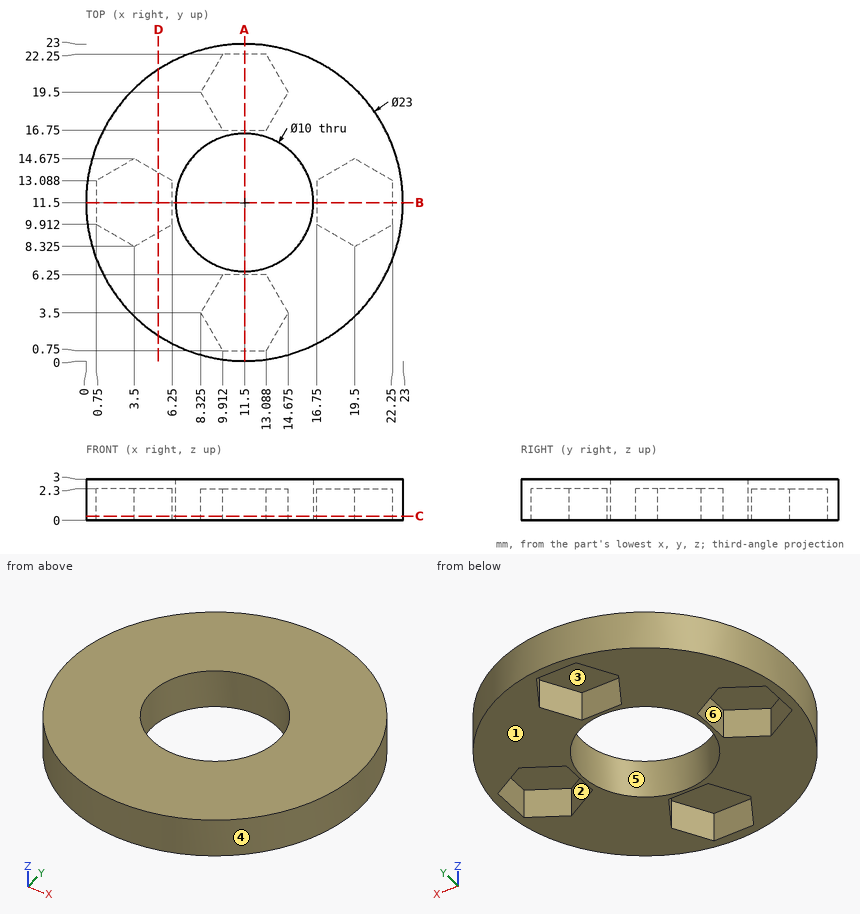
Design review of the part shown in the three views and the two pictorial views. Dimensions are in mm from the part's minimum x, y and z. A direction names the side the tool comes from. Round coordinates to 2 decimals unless told otherwise and drop trailing zeros. Write each loop counter-clockwise with the first axis right and the second up, starting at its lowest first coordinate (ties: lowest second). Pieces come first, ordered by that corner, then holes. Notation, with made-up numbers: (86, -34.5) -> (139, -34.5) arc R32 ccw to (139, -2.5) -> close; hole circle Ø2 at (-3.75, -21). An arc over 180 degrees is marked (long way). One line per question, with ' | ' between items. Start each with the question number.
1) Add section D-D (x = 5.25). Write out the cut boundary in (y, z) (1 decimal).
2) Add section C-C (z = 0.3). Count the separate pieces of the cut face and the enclosed holes in it, and give its area (3 significant figures).
3) Machinability: for the marked faces 5 and 6, which of the approach directions +Z, -Z, +X, -X, +Y, -Y give a long, thin tool a straight path to every point of the face, cutting with its end or side? Answer none if there is none.
4) Mouldability with a two-part tool opening along X and no side actions: class the marked faces 1, 2, 3 and 4 as +X half, -X half, draft (parallel to the pull), parting line (faces both ways), or undercut.
5) For pin 1 Ø1.6 at (x, y) = (3.5, 11.5) entering from -Z; pin 2 Ø0.7 at (y, z) = (11, 1.5) entering from -X, all flat-tipped, find the tip position at first contact; note any pin that passes through.
6) Add section A-A (x = 11.5). Write out the cut boundary in (y, z).
7) Wall thickness on line 1 along Y through (x, z) = (11.75, 0.25); line 2 along Y through (x, z) = (12.5, 1.55); line 3 along X through (y, z) = (13.5, 0.95) (1 decimal): over which ranges is each line inside the solid? List them lowest first.
Reported:
1) outline: (1.8, 0) -> (9.3, 0) -> (9.3, 2.3) -> (13.7, 2.3) -> (13.7, 0) -> (21.2, 0) -> (21.2, 3) -> (1.8, 3) -> close
2) separate pieces: 1 | enclosed holes: 5 | area: 232 mm²
3) face 5: +Z, -Z | face 6: -Z
4) face 1: draft | face 2: undercut | face 3: undercut | face 4: parting line
5) pin 1: stops at z = 2.3 | pin 2: stops at x = 0
6) outline: (0, 0) -> (0.75, 0) -> (0.75, 2.3) -> (6.25, 2.3) -> (6.25, 0) -> (6.5, 0) -> (6.5, 3) -> (0, 3) -> close; (16.5, 0) -> (16.75, 0) -> (16.75, 2.3) -> (22.25, 2.3) -> (22.25, 0) -> (23, 0) -> (23, 3) -> (16.5, 3) -> close
7) line 1: y = 0 to 0.75, 6.25 to 6.51, 16.49 to 16.75, 22.25 to 23 | line 2: y = 0.04 to 0.75, 6.25 to 6.6, 16.4 to 16.75, 22.25 to 22.96 | line 3: x = 0.2 to 1.5, 5.5 to 6.9, 16.1 to 17.5, 21.5 to 22.8
